```python
from build123d import *

# Parameters (mm, degrees)
SKETCH2_W           = 63.5
SKETCH2_H           = 63.5
SKETCH2_R           = 26.19375
BOSS_EXTRUDE1_DEPTH = 279.4
BOSS_EXTRUDE2_START = -12.7
SKETCH3_W           = 88.9
SKETCH3_H           = 88.9
SKETCH3_R           = 26.19375
BOSS_EXTRUDE2_DEPTH = 12.7
SKETCH4_W           = 63.5
SKETCH4_H           = 63.5
SKETCH4_R           = 23.114
BOSS_EXTRUDE3_DEPTH = 12.7
SKETCH5_R           = 23.114
SKETCH5_R_2         = 19.05
BOSS_EXTRUDE4_DEPTH = 6.35
CUT_EXTRUDE4_START  = -76.2
CUT_EXTRUDE4_DEPTH  = 88.9


# Read off the part's stored shape, not the designer's step: Cut-Extrude4
with BuildPart() as part:
    # Sketch2 → Boss-Extrude1 (new body)
    with BuildSketch(Plane.XY):
        with Locations((31.75, 31.75)):
            Rectangle(SKETCH2_W, SKETCH2_H)
        with Locations((31.75, 31.75)):
            Circle(SKETCH2_R, mode=Mode.SUBTRACT)
    extrude(amount=BOSS_EXTRUDE1_DEPTH)

    # Sketch3 → Boss-Extrude2 (add)
    with BuildSketch(Plane.XY.offset(279.4).offset(BOSS_EXTRUDE2_START)):
        with Locations((31.75, 31.75)):
            Rectangle(SKETCH3_W, SKETCH3_H)
        with Locations((31.75, 31.75)):
            Circle(SKETCH3_R, mode=Mode.SUBTRACT)
    extrude(amount=BOSS_EXTRUDE2_DEPTH)

    # Sketch4 → Boss-Extrude3 (add)
    with BuildSketch(Plane(origin=(0, 0, 0), x_dir=(-1, 0, 0), z_dir=(0, 0, -1))):
        with Locations((-31.75, 31.75)):
            Rectangle(SKETCH4_W, SKETCH4_H)
        with Locations((-31.75, 31.75)):
            Circle(SKETCH4_R, mode=Mode.SUBTRACT)
    extrude(amount=BOSS_EXTRUDE3_DEPTH)


with BuildPart() as body_2:
    # Sketch5 → Boss-Extrude4 (new body)
    with BuildSketch(Plane(origin=(0, 0, -6.35), x_dir=(-1, 0, 0), z_dir=(0, 0, -1))):
        with Locations((-31.75, 31.75)):
            Circle(SKETCH5_R)
        with Locations((-31.75, 31.75)):
            Circle(SKETCH5_R_2, mode=Mode.SUBTRACT)
    extrude(amount=-BOSS_EXTRUDE4_DEPTH)


with BuildPart() as cut_extrude4_tool:
    # Cut-Extrude4 outline → Cut-Extrude4 (new body)
    with BuildSketch(Plane(origin=(63.5, 0, 0), x_dir=(0, 0, -1), z_dir=(1, 0, 0)).offset(CUT_EXTRUDE4_START)):
        Polygon((-266.7, 44.45), (-266.7, 76.2), (-279.4, 76.2), (-279.4, -12.7), (-266.7, -12.7), (-266.7, 0), (12.7, 0), (12.7, 63.5), (0, 63.5), (0, 44.45), align=None)
    extrude(amount=CUT_EXTRUDE4_DEPTH)


with BuildPart() as part_1:
    add(part.part)

    # Cut-Extrude4: cut by cut_extrude4_tool
    add(cut_extrude4_tool.part, mode=Mode.SUBTRACT)


with BuildPart() as body_2_1:
    add(body_2.part)

    # Cut-Extrude4: cut by cut_extrude4_tool
    add(cut_extrude4_tool.part, mode=Mode.SUBTRACT)


solid = part_1.part
```
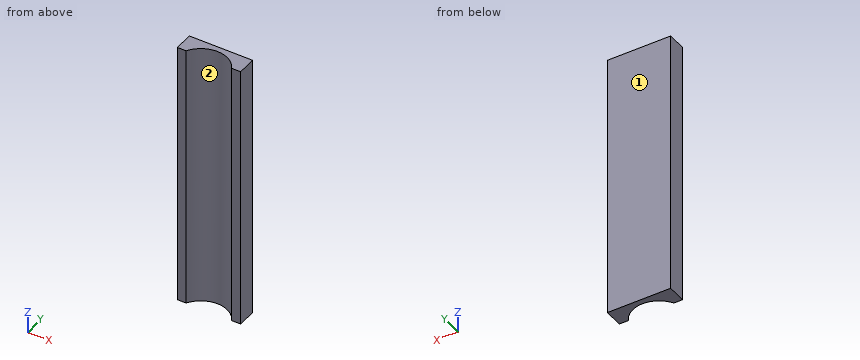
The model under review builds one solid part; all positions refer to its coordinate system, in mm. Face numbers are marked on the shaded views. Round coordinates to 2 decimals unless told otherwise and drop trailing zeros. Order: outer loops, then holes, each group sorted by start corner. A loop starts at its lowest first (then second) coordinate and runs counter-clockwise, first axis right, second up. Notation, with made-up numbers: (72, 20.5) - (87, 20.5) arc R23 cw to (87, 44.5) - close; hole circle Ø10 at (-10, 76.5). An arc over 180 degrees is marked (long way). Answer in a Markdown table with one row per item.
(1) Take a section at B-B on z = 77. Write out the cut boundary in (x, y).
Result set:
| item | result |
|---|---|
| outline | (0, 44.45) - (8.84, 44.45) arc R26.19 cw to (54.66, 44.45) - (63.5, 44.45) - (63.5, 63.5) - (0, 63.5) - close |
(2) Take a section at A-A on y = 48.25. Write out the cut boundary in (x, z), plus the area to 3 significant figures.
Result set:
| item | result |
|---|---|
| outline | (0, 0) - (11.41, 0) - (11.41, 266.7) - (0, 266.7) - close; (52.09, 0) - (63.5, 0) - (63.5, 266.7) - (52.09, 266.7) - close |
| area | 6,080 mm2 |
(3) For line 1 (X direction, y = 51, z = 92); line 2 (Y direction, x = 31, z = 190); line 3 (X direction, y = 55.75, z = 142.5), list the stretches that pass through material, from the lowest coordinate up. Write a range as from..to.
Result set:
| item | result |
|---|---|
| line 1 | x = 0..13.99, 49.51..63.5 |
| line 2 | y = 57.93..63.5 |
| line 3 | x = 0..21.26, 42.24..63.5 |
(4) Take a section at D-D on x = 52. Write out the cut boundary in (y, z).
Result set:
| item | result |
|---|---|
| outline | (48.36, 0) - (63.5, 0) - (63.5, 266.7) - (48.36, 266.7) - close |
(5) Mouldability with a two-part tool opening along X and no side actions: class the marked faces 1 and 2 as released by +X, released by -X, zero draft, split by the parting line, or undercut.
Result set:
| item | result |
|---|---|
| face 1 | zero draft |
| face 2 | undercut |
(6) Clearance check with a flat-ended pin moving along its axis: P1, Ø8, axis at x = 15.5, z = 117, coming from the -Y side. State where the tip first meets the part, or that it passes through.
Result set:
| item | result |
|---|---|
| P1 | stops at y = 48.36 |
(7) Take a section at C-C on x = 28. Write out the cut boundary in (y, z), plus the area to 3 significant figures.
Result set:
| item | result |
|---|---|
| outline | (57.67, 0) - (63.5, 0) - (63.5, 266.7) - (57.67, 266.7) - close |
| area | 1,550 mm2 |
